Input: part model. Units: mm. Frame: model coordinates. Face numbers are marked on the shaded views. Round coordinates to 2 decimals unless told otherwise and drop trailing zeros. Write each loop counter-clockwise with the first axis right and the second up, starting at its lowest first coordinate (ties: lowest second). Pieces come first, ordered by that corner, then holes. Notation, with made-up numbers: (82, -5.5) -> (116, -5.5) arc R32 cw to (116, 25.5) -> close; hole circle Ø3 at (37, 64). An arc over 180 degrees is marked (long way). Write item = value, one per line.
Autodesk Inventor part; units mm, degrees
sketch "Boceto1" plane through (0, 0, 0) normal (0, 0, 1) x (1, 0, 0)
  line L0 (-75, 75) -> (75, 75)
  line L1 (75, 75) -> (75, -75)
  line L2 (75, -75) -> (-75, -75)
  line L3 (-75, -75) -> (-75, 75)
  line L4 (-75, 75) -> (75, -75) construction
  line L5 (75, 75) -> (-75, -75) construction
  point P0 (0, 0)
  dimension "d0" = 150
  dimension "d1" = 150
extrude "Extrusión1" add sketch "Boceto1" along normal blind 25.4
sketch "Boceto2" plane through (75, -75, 0) normal (1, 0, 0) x (0, 0, -1)
  line L0 (-25.4, 150) -> (-25.4, 0)
  line L1 (-25.4, 0) -> (-25.4, 150)
  line L2 (-25.4, 75) -> (-25.4, 60)
  line L3 (-25.4, 75) -> (-10.4, 75)
  line L4 (-10.4, 75) -> (-25.4, 60)
  line L5 (-25.4, 75) -> (-25.4, 90)
  line L6 (-25.4, 90) -> (-10.4, 75)
  point P0 (0, 75)
  dimension "d6" = 15
  dimension "d7" = 15
  dimension "d9" = 15
extrude "Extrusión2" cut sketch "Boceto2" against normal blind 165.25
fillet "Empalme1" radius 7 1 edges at (0, 0, 10.4)
properties part number "Placa - Grieta"
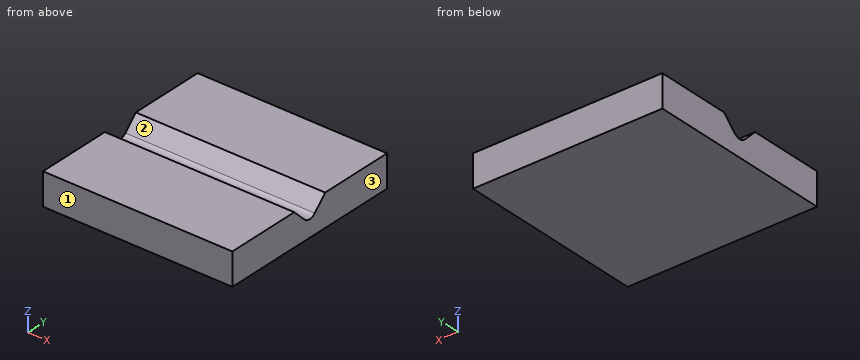
1) Line query: L1, parallel to Y at x = 54, z = 17.75; L2, parallel to Y at x = 30, z = 20.5; L3, parallel to Z at x = 4.5, y = -12. Output: solid intervals per line, ascending. Write a range as from..to.
Solutions:
L1 = -75..-7.35, 7.35..75
L2 = -75..-10.1, 10.1..75
L3 = 0..22.4
2) Cut plane B-B (x = 12). Return the cut outline in (y, z).
Solutions:
outline = (-75, 0) -> (75, 0) -> (75, 25.4) -> (15, 25.4) -> (4.95, 15.35) arc R7 cw to (-4.95, 15.35) -> (-15, 25.4) -> (-75, 25.4) -> close
3) Cut plane A-A (z = 23.5). Return the cut outline in (x, y).
Solutions:
outline = (-75, -75) -> (75, -75) -> (75, -13.1) -> (-75, -13.1) -> close; (-75, 13.1) -> (75, 13.1) -> (75, 75) -> (-75, 75) -> close
4) Draft query along Y for the marked faces 1, 2 and 3. Return one class per face: +Y half, -Y half, draft (parallel to the pull), parting line (faces both ways), or undercut.
Solutions:
face_1 = -Y half
face_2 = undercut
face_3 = draft
5) Cut plane C-C (y = -9). Return the cut outline in (x, z).
Solutions:
outline = (-75, 0) -> (75, 0) -> (75, 19.4) -> (-75, 19.4) -> close
